```python
from build123d import *

# Parameters (mm, degrees)
F1_DEPTH = 17.5
F4_T     = -2
F6_D     = 6


with BuildPart() as f1:
    # F0 (on Top) → F1 (new body, symmetric)
    with BuildSketch(Plane.XY):
        Polygon((0, 0), (0, 17.5), (-180, 17.5), (-180, 260), (-215, 260), (-215, 0), align=None)
    extrude(amount=F1_DEPTH, both=True)

    # F2: F1 across plane


with BuildPart() as f1_1:
    add(f1.part)
    add(f1.part.mirror(Plane.XZ))

    # F3: F1 across plane


with BuildPart() as f1_2:
    add(f1_1.part)
    add(f1_1.part.mirror(Plane.YZ))

    # F4
    f4_openings = [f1_2.faces().sort_by_distance(p)[0] for p in [
        (-197.5, -260, 0),
        (197.5, -260, 0),
        (197.5, 260, 0),
        (-197.5, 260, 0),
    ]]
    offset(amount=F4_T, openings=f4_openings, kind=Kind.INTERSECTION)

    # F6 (through all)
    with Locations(Plane.XY.offset(17.5)):
        with Locations((-68, 0), (-58.5, 7.5), (-49, 0), (-58.5, -7.5)):
            Hole(F6_D / 2)


solid = f1_2.part
```
The listing builds one solid part. Answer for the finished solid, in the listing's coordinates (mm). A direction names the side the tool comes from. Round coordinates to 2 decimals unless told otherwise and drop trailing zeros. Loops run counter-clockwise (first coordinate to the right, second up) from the corner with the lowest first, then second, coordinate; pieces in that order, holes last. Notation, with made-up numbers: (39.25, 63) - (80.25, 63) arc R13 cw to (80.25, 73) - close; hole circle Ø8 at (-40, -16). An arc over 180 degrees is marked (long way). Return JSON: item names as keys, results as strings. Group by question number.
1. Consider probe 1 along X at (y, z) = (-102, -7); probe 2 along Y at (x, z) = (-58.5, 16.2); probe 3 along Y at (x, z) = (119, 10.5). Determine where each line is inside the solid, lowest interval first.
2. The part is cut by section C-C on x = 95. Determine the outline of the cut face in (y, z).
3. Each of these flat-tipped pins is pushed along its axis until it touches: P1, Ø3.5, axis at x = -58.5, y = 7.5, coming from the -Z side; P2, Ø17.5, axis at x = 0.5, z = 8, coming from the +Y side. Where does it stop, or does it pass through?
4. Which of the six approach directions +Z, -Z, +X, -X, +Y, -Y give full straight-line access (tool end or side, diameter ignored) to faces 1 (the flat face through (1, -1, 15.5)), 2 (the flat face through (213, -4, 0)), 3 (the flat face through (180, -137, 0)), 4 (the flat face through (-180, 137, 0))?
5. The part is cut by section B-B on z = 2. Determine the outline of the cut face in (x, y), then the cut area to 3 significant figures.
6. The part is cut by section A-A on y = -192. Determine the outline of the cut face in (x, z).
7. The mould has two halves that part along Z. Classify faces 5 (the flat face through (1, -1, 17.5)), 6 (the flat face through (-196, -260, 16)), 7 (the flat face through (-182, 136, 0)): pulls with the +Z half, pulls with the -Z half, needs draft (parallel to the pull), parting line crosses it, or undercut.
Resolved:
{
 "1": {"probe 1": "x = -215 to -213, -182 to -180, 180 to 182, 213 to 215", "probe 2": "y = -17.5 to -10.5, -4.5 to 4.5, 10.5 to 17.5", "probe 3": "y = -17.5 to -15.5, 15.5 to 17.5"},
 "2": {"outline": "(-17.5, -17.5) - (17.5, -17.5) - (17.5, 17.5) - (-17.5, 17.5) - close; hole (-15.5, -15.5) - (15.5, -15.5) - (15.5, 15.5) - (-15.5, 15.5) - close"},
 "3": {"P1": "passes through", "P2": "stops at y = 17.5"},
 "4": {"face 1": "none", "face 2": "+Y, -Y", "face 3": "+Z, -Z, -Y", "face 4": "+Z, -Z, +Y"},
 "5": {"outline": "(-215, -260) - (-213, -260) - (-213, 260) - (-215, 260) - close; (-182, -260) - (-180, -260) - (-180, -17.5) - (180, -17.5) - (180, -260) - (182, -260) - (182, -15.5) - (-182, -15.5) - close; (-182, 15.5) - (182, 15.5) - (182, 260) - (180, 260) - (180, 17.5) - (-180, 17.5) - (-180, 260) - (-182, 260) - close; (213, -260) - (215, -260) - (215, 260) - (213, 260) - close", "area": "5,480 mm²"},
 "6": {"outline": "(-215, -17.5) - (-180, -17.5) - (-180, 17.5) - (-215, 17.5) - close; (180, -17.5) - (215, -17.5) - (215, 17.5) - (180, 17.5) - close; hole (-213, -15.5) - (-182, -15.5) - (-182, 15.5) - (-213, 15.5) - close; hole (182, -15.5) - (213, -15.5) - (213, 15.5) - (182, 15.5) - close"},
 "7": {"face 5": "pulls with the +Z half", "face 6": "needs draft", "face 7": "undercut"}
}
